```python
from build123d import *

# Parameters (mm, degrees)
R_VOL_MINCE1_OUTLINE_W = 0.5
R_VOL_MINCE1_OUTLINE_H = 1
CONG_2_R               = 10
CONG_3_R               = 10


# Read off the part's stored shape, not the designer's step: Révol.-Mince1
with BuildPart() as part:
    # Révol.-Mince1 outline → Révol.-Mince1 (revolve)
    with BuildSketch(Plane.XY):
        Polygon((2.5, 5), (2.5, 0), (7, 0), (7, 28), (31.169797205, 28), (34.60776491, 0), (40.254430878, 0), (40.254430878, 3), (36.254430878, 3), (32.939247734, 30), (5, 30), (5, 5), align=None)
        with Locations((4.75, 2.5)):
            Rectangle(R_VOL_MINCE1_OUTLINE_W, R_VOL_MINCE1_OUTLINE_H, mode=Mode.SUBTRACT)
    revolve(axis=Axis((0, 0, 0), (0, 1, 0)))

    # Congé2
    cong_2_edges = [part.edges().sort_by_distance(p)[0] for p in [
        (-31.169797205, 28, 0),
    ]]
    fillet(cong_2_edges, radius=CONG_2_R)

    # Congé3
    cong_3_edges = [part.edges().sort_by_distance(p)[0] for p in [
        (-7, 28, 0),
    ]]
    fillet(cong_3_edges, radius=CONG_3_R)


solid = part.part
```
The listing builds one solid part. Answer for the finished solid, in the listing's coordinates (mm). A direction names the side the tool comes from. Give positions to 0.01 mm unless a question says otherwise; leave off trailing zeros. Write each loop counter-clockwise with the first axis right and the second up, starting at its lowest first coordinate (ties: lowest second). Pieces come first, ordered by that corner, then holes. Notation, with made-up numbers: (56.25, -40) -> (98.25, -40) arc R19 ccw to (98.25, -17) -> close; hole circle Ø11 at (73.5, 31.5). An arc over 180 degrees is marked (long way). Write item = value, one per line. Start each with the question number.
1) Each of these flat-tipped pins is pushed along its axis until it touches: pin 1 (1 mm diameter, centred on y = 25.5, z = 25.5, fed in from +X); pin 2 (6.5 mm diameter, centred on x = 0, z = 0, fed in from +Y); pin 3 (10 mm diameter, centred on y = 7.5, z = -10, fed in from +X). Where does it stop, or does it pass through?
2) The part is cut by section A-A, the plane x = 0. Count the separate pieces of the cut face and the enclosed holes in it, and give its area (3 significant figures).
3) Which of the six approach directions +Z, -Z, +X, -X, +Y, -Y give full straight-line access (tool end or side, diameter ignored) to faces 4 (the face through (-36, 3, -6)), 5 (the face through (-18, 0, -30)), 6 (the face through (5.1, 28, 16.4)), 7 (the face through (-1.08, 2.51, 4.88))?
4) Determine the mould class of faces 1 (the face through (38.396, 1.521, -12.091)), 2 (the face through (-26.124, 13.746, 20.031)), 3 (the face through (0, 30, 7)) for opening direction Z: +Z half, -Z half, draft (parallel to the pull), parting line (faces both ways), or undercut.
5) The part is cut by section C-C, the plane y = 21. Determine the outline of the cut face in (x, z), and give its area (3 significant figures).
6) Straight lines are drawn through the part: line 1 along X through (y, z) = (10, 2.5); line 2 along Z through (x, y) = (0, 21); line 3 along Z through (x, y) = (-4, 15). For each, find the intervals that lie inside material, in ascending order.
7) The part is cut by section D-D, the plane y = 7.5. Determine the outline of the cut face in (x, z), and give its area (3 significant figures).
Solutions:
q1.pin_1 = 22.29
q1.pin_2 = 5
q1.pin_3 = 39.49
q2.separate_pieces = 2
q2.enclosed_holes = 2
q2.area = 459 mm²
q3.face_4 = +Y
q3.face_5 = +Z, -Z, +X, -X, -Y
q3.face_6 = -Y
q3.face_7 = none
q4.face_1 = parting line
q4.face_2 = undercut
q4.face_3 = draft
q5.outline = circle Ø68.09 at (0, 0); circle Ø14.92 at (0, 0); hole circle Ø63.72 at (0, 0); hole circle Ø10 at (0, 0)
q5.area = 548 mm²
q6.line_1 = -35.31 to -33.29, -6.54 to -4.33, 4.33 to 6.54, 33.29 to 35.31
q6.line_2 = -34.04 to -31.86, -7.46 to -5, 5 to 7.46, 31.86 to 34.04
q6.line_3 = -34.55 to -32.52, -5.74 to -3, 3 to 5.74, 32.52 to 34.55
q7.outline = circle Ø71.4 at (0, 0); circle Ø14 at (0, 0); hole circle Ø67.37 at (0, 0); hole circle Ø10 at (0, 0)
q7.area = 515 mm²
